Geometry check sheet. Reference: drawing and pictorial views, mm from the part's lowest x, y, z. A direction names the side the tool comes from. Round coordinates to 2 decimals unless told otherwise and drop trailing zeros. Loops run counter-clockwise (first coordinate to the right, second up) from the corner with the lowest first, then second, coordinate; pieces in that order, holes last. Notation, with made-up numbers: (10.5, 8) - (28.5, 8) arc R18 cw to (28.5, 18) - close; hole circle Ø5 at (-35.5, 27). An arc over 180 degrees is marked (long way). Return JSON: item names as keys, results as strings.
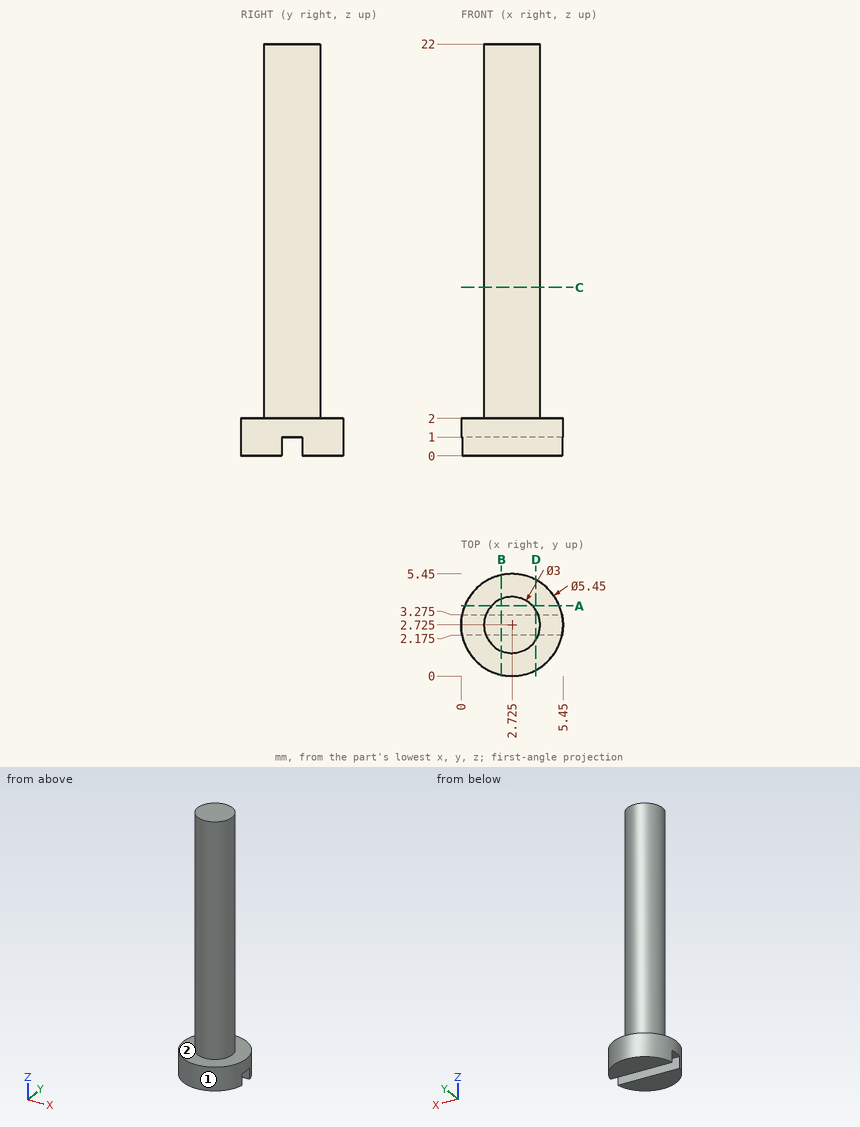
Q1. Sectioned sample at C-C (z = 9). Enter the section's corners in (x, y) (3 decimals).
Answer key:
{"outline": "circle Ø3 at (2.725, 2.725)"}
Q2. Sectioned sample at A-A (y = 3.75). Enter the section's corners in (x, z).
Answer key:
{"outline": "(0.2, 0) - (5.25, 0) - (5.25, 2) - (3.82, 2) - (3.82, 22) - (1.63, 22) - (1.63, 2) - (0.2, 2) - close"}
Q3. Sectioned sample at B-B (x = 2.15). Enter the section's corners in (y, z) (3 decimals).
Answer key:
{"outline": "(0.061, 0) - (2.175, 0) - (2.175, 1) - (3.275, 1) - (3.275, 0) - (5.389, 0) - (5.389, 2) - (4.11, 2) - (4.11, 22) - (1.34, 22) - (1.34, 2) - (0.061, 2) - close"}
Q4. Sectioned sample at D-D (x = 4). Enter the section's corners in (y, z) (3 decimals), plus the area to 3 significant figures.
Answer key:
{"outline": "(0.317, 0) - (2.175, 0) - (2.175, 1) - (3.275, 1) - (3.275, 0) - (5.133, 0) - (5.133, 2) - (3.515, 2) - (3.515, 22) - (1.935, 22) - (1.935, 2) - (0.317, 2) - close", "area": "40.1 mm²"}
Q5. Depth check by flat-ended pin: P1, Ø1, axis at x = 2.5, z = 10, coming from the -Y side (3 decimals); P2, Ø1, axis at x = 2, z = 4.5, coming from the +Y side. Enter the tip coordinate at first touch or a pass-through.
Answer key:
{"P1": "stops at y = 1.225", "P2": "stops at y = 4.21"}
Q6. Tool access check on the marked faces 1 and 2. Record the directions out of +Z, -Z, +X, -X, +Y, -Y that give a thin tool (end or side, any length) a straight path to the whole face; none if there is none.
Answer key:
{"face 1": "+Z, -Z", "face 2": "+Z"}
Q7. Scan lines: probe 1 along Z at (x, y) = (4.5, 4.05); probe 2 along X at (y, z) = (2.85, 15.5); probe 3 along Z at (x, y) = (3.3, 2.5). Record each from-to range of solid material in increasing order. Write a range as [from, to].
Answer key:
{"probe 1": "z = [0, 2]", "probe 2": "x = [1.23, 4.22]", "probe 3": "z = [1, 22]"}
